Geometry: final body of the model. Coordinates: model frame, mm. A direction names the side the tool comes from. Give positions to 0.01 mm unless a question says otherwise; leave off trailing zeros. Write each loop counter-clockwise with the first axis right and the second up, starting at its lowest first coordinate (ties: lowest second). Pieces come first, ordered by that corner, then holes. Notation, with made-up numbers: (69.5, 30.5) -> (82.5, 30.5) arc R16 cw to (82.5, 57.5) -> close; hole circle Ø3 at (2.5, 42.5). An arc over 180 degrees is marked (long way). Answer as a JSON object with one key per item and string values.
from build123d import *

# Parameters (mm, degrees)
PROFILEEXTRUDE_DEPTH = 73.76
HOSEWINDOW_W         = 16.29
HOSEWINDOW_H         = 26.5
HOSEWINDOWCUT_DEPTH  = 22.63
CAGESCREWS_R         = 2.4
CAGESCREWSCUT_DEPTH  = 22.63
AXLEHOLECUT_DEPTH    = 22.63
SETSCREWS_R          = 2.426338021
SETSCREWS_R_2        = 2.788762315
SETSCREWSCUT_DEPTH   = 22.63
SKETCH1_W            = 6.7
SKETCH1_H            = 6.7
CUT_EXTRUDE1_DEPTH   = 22.63
FILLET1_R            = 1


with BuildPart() as part:
    # Profile → ProfileExtrude (new body)
    with BuildSketch(Plane.XY):
        with BuildLine():
            Line((-6.44073477, -58.62791746), (-6.44073477, -33.62791746))
            Line((-6.44073477, -33.62791746), (4.13926523, -33.62791746))
            Line((4.13926523, -33.62791746), (4.13926523, -18.13791746))
            ThreePointArc((4.13926523, -18.13791746), (7.563334043, -14.326029686), (9.63126523, -9.63791746))
            Line((9.63126523, -9.63791746), (11.94926523, -9.63791746))
            Line((11.94926523, -9.63791746), (11.94926523, 0.36208254))
            Line((11.94926523, 0.36208254), (9.62926523, 0.36208254))
            ThreePointArc((9.62926523, 0.36208254), (7.643946533, 4.440626184), (4.60926523, 7.81208254))
            Line((4.60926523, 7.81208254), (4.60926523, 17.41208254))
            Line((4.60926523, 17.41208254), (-6.44073477, 17.41208254))
            Line((-6.44073477, 17.41208254), (-6.44073477, 27.41208254))
            Line((-6.44073477, 27.41208254), (15.18926523, 27.41208254))
            Line((15.18926523, 27.41208254), (15.18926523, -58.62791746))
            Line((15.18926523, -58.62791746), (-6.44073477, -58.62791746))
        make_face()
    extrude(amount=PROFILEEXTRUDE_DEPTH)

    # HoseWindow → HoseWindowCut (cut, through all)
    with BuildSketch(Plane(origin=(15.18926523, 0, 0), x_dir=(0, 0, -1), z_dir=(1, 0, 0))):
        with Locations((-56.725, -45.37791746)):
            Rectangle(HOSEWINDOW_W, HOSEWINDOW_H)
    extrude(amount=-HOSEWINDOWCUT_DEPTH, mode=Mode.SUBTRACT)

    # CageScrews → CageScrewsCut (cut, through all)
    with BuildSketch(Plane(origin=(15.18926523, 0, 0), x_dir=(0, 0, -1), z_dir=(1, 0, 0))):
        with Locations((-66.26, 22.41208254)):
            Circle(CAGESCREWS_R)
        with Locations((-7.5, 22.41208254)):
            Circle(CAGESCREWS_R)
        with Locations((-7.5, -53.62791746)):
            Circle(CAGESCREWS_R)
        with Locations((-69.31, -53.62791746)):
            Circle(CAGESCREWS_R)
    extrude(amount=-CAGESCREWSCUT_DEPTH, mode=Mode.SUBTRACT)

    # AxleHole → AxleHoleCut (cut, through all)
    with BuildSketch(Plane(origin=(15.18926523, 0, 0), x_dir=(0, 0, -1), z_dir=(1, 0, 0))):
        with BuildLine():
            Line((-44.699, 2.307293484), (-47.361, 2.307293484))
            Line((-47.361, 2.307293484), (-47.361, 3.926293484))
            ThreePointArc((-47.361, 3.926293484), (-46.03, -9.21691746), (-44.699, 3.926293484))
            Line((-44.699, 3.926293484), (-44.699, 2.307293484))
        make_face()
    extrude(amount=-AXLEHOLECUT_DEPTH, mode=Mode.SUBTRACT)

    # SetScrews → SetScrewsCut (cut, through all)
    with BuildSketch(Plane(origin=(15.18926523, 0, 0), x_dir=(0, 0, -1), z_dir=(1, 0, 0))):
        with Locations((-85.624962528, 3.100017238)):
            Circle(SETSCREWS_R)
        with Locations((-24.037149362, -2.017095907)):
            Circle(SETSCREWS_R_2)
    extrude(amount=-SETSCREWSCUT_DEPTH, mode=Mode.SUBTRACT)

    # Sketch1 → Cut-Extrude1 (cut, through all)
    with BuildSketch(Plane(origin=(15.18926523, 0, 0), x_dir=(0, 0, -1), z_dir=(1, 0, 0))):
        with Locations((-18.35, -48.92791746)):
            Rectangle(SKETCH1_W, SKETCH1_H)
        with Locations((-30.95, -48.92791746)):
            Rectangle(SKETCH1_W, SKETCH1_H)
        with Locations((-5.75, -36.22791746)):
            Rectangle(SKETCH1_W, SKETCH1_H)
        with Locations((-18.35, -36.22791746)):
            Rectangle(SKETCH1_W, SKETCH1_H)
        with Locations((-5.75, -21.22791746)):
            Rectangle(SKETCH1_W, SKETCH1_H)
        with Locations((-18.35, -21.22791746)):
            Rectangle(SKETCH1_W, SKETCH1_H)
    extrude(amount=-CUT_EXTRUDE1_DEPTH, mode=Mode.SUBTRACT)

    # Fillet1
    fillet1_edges = [part.edges().sort_by_distance(p)[0] for p in [
        (15.18926523, -45.57791746, 18.35),
        (15.18926523, -48.92791746, 21.7),
        (15.18926523, -52.27791746, 18.35),
        (15.18926523, -48.92791746, 15),
        (15.18926523, -48.92791746, 34.3),
        (15.18926523, -52.27791746, 30.95),
        (15.18926523, -48.92791746, 27.6),
        (15.18926523, -45.57791746, 30.95),
        (15.18926523, -36.22791746, 9.1),
        (15.18926523, -39.57791746, 5.75),
        (15.18926523, -36.22791746, 2.4),
        (15.18926523, -32.87791746, 5.75),
        (15.18926523, -36.22791746, 21.7),
        (15.18926523, -39.57791746, 18.35),
        (15.18926523, -36.22791746, 15),
        (15.18926523, -32.87791746, 18.35),
        (15.18926523, -15.60791746, 0),
        (15.18926523, -21.22791746, 9.1),
        (15.18926523, -24.57791746, 5.75),
        (15.18926523, -21.22791746, 2.4),
        (15.18926523, -17.87791746, 5.75),
        (15.18926523, -21.22791746, 21.7),
        (15.18926523, -24.57791746, 18.35),
        (15.18926523, -21.22791746, 15),
        (15.18926523, -17.87791746, 18.35),
        (15.18926523, -58.62791746, 69.315),
        (15.18926523, 27.41208254, 36.88),
        (15.18926523, -58.62791746, 24.29),
        (15.18926523, -15.60791746, 73.76),
        (15.18926523, -45.37791746, 64.87),
        (15.18926523, -45.37791746, 48.58),
        (15.18926523, -32.12791746, 56.725),
    ]]
    fillet(fillet1_edges, radius=FILLET1_R)


solid = part.part
Q1. Mould query, pull axis Z, two halves, no side actions, for faces 1 (the flat face through (4, -39.578, 6)), 2 (the flat face through (11.949, -5, 36)). Classes: pulls with the +Z half, pulls with the -Z half, needs draft (parallel to the pull), parting line crosses it, or undercut.
Values:
{"face 1": "undercut", "face 2": "needs draft"}
Q2. First-contact query: P1, Ø2, axis at y = -5.5, z = 57.5, coming from the -X side; P2, Ø6, axis at y = -29, z = 48.5, coming from the -X side; P3, Ø4, axis at y = 3.5, z = 59.5, coming from the -X side. Flat tips, straight axial feed; report the tip coordinate or a pass-through.
Values:
{"P1": "x = 11.95", "P2": "x = 4.14", "P3": "x = 6.87"}
Q3. Set-up query: faces 3 (the flat face through (4, -49, 27.6)), 4 (the flat face through (4, -46, 64.87)), 5 (the flat face through (-1, 17.412, 36)). Return all of +Z, -Z, +X, -X, +Y, -Y with unobstructed straight access to the full face (end or side cutting, diameter ignored); none if empty.
Values:
{"face 3": "+X, -X", "face 4": "+X, -X, -Y", "face 5": "+Z, -Z, -X"}
Q4. Cut plane A-A (z = 46.03). Return the cut outline in (x, y).
Values:
{"outline": "(-6.44, -58.63) -> (14.19, -58.63) arc R1 ccw to (15.19, -57.63) -> (15.19, -9.22) -> (11.95, -9.22) -> (11.95, -9.64) -> (9.63, -9.64) arc R16.26 cw to (4.14, -18.14) -> (4.14, -33.63) -> (-6.44, -33.63) -> close; (-6.44, 17.41) -> (4.61, 17.41) -> (4.61, 7.81) arc R16.26 cw to (8.86, 2.31) -> (15.19, 2.31) -> (15.19, 26.41) arc R1 ccw to (14.19, 27.41) -> (-6.44, 27.41) -> close"}
Q5. Cut plane D-D (y = -27.5). Return the cut outline in (x, z), and give its area (3 significant figures).
Values:
{"outline": "(4.14, 0) -> (14.19, 0) arc R1 ccw to (15.19, 1) -> (15.19, 72.76) arc R1 ccw to (14.19, 73.76) -> (4.14, 73.76) -> close", "area": "815 mm²"}
Q6. Cut plane B-B (x = 1.5). State how many separate pieces and enclosed holes the cut face has, and give its area (3 significant figures).
Values:
{"separate pieces": "3", "enclosed holes": "6", "area": "1,930 mm²"}
Q7. Material intervals for L1, parallel to Y at x = 0.5, z = 30; L2, parallel to Y at x = 4.25, z = 7.5; L3, parallel to Z at x = 11.25, y = -20, sorted ascending. Write a range as from..to.
Values:
{"L1": "-58.63..-52.28, -45.58..-33.63, 17.41..27.41", "L2": "-58.63..-56.03, -51.23..-39.58, -32.88..-24.58, 17.41..20.01, 24.81..27.41", "L3": "0..2.4, 9.1..15, 21.7..73.76"}
